from build123d import *

# Parameters (mm, degrees)
SKETCH_1_R      = 2
EXTRUDE_1_DEPTH = 3


with BuildPart() as part:
    # 草图1 → 凸台-拉伸1 (new body)
    with BuildSketch(Plane.XY):
        with BuildLine():
            Line((47.983882687, 10.173144913), (30.663374611, 20.173144913))
            ThreePointArc((30.663374611, 20.173144913), (-1.771986525, 14.862979702), (-28.921960456, 33.386732619))
            Line((-28.921960456, 33.386732619), (-48.921960456, 33.386732619))
            Line((-48.921960456, 33.386732619), (-48.921960456, -16.613267381))
            Line((-48.921960456, -16.613267381), (-28.921960456, -16.613267381))
            ThreePointArc((-28.921960456, -16.613267381), (-22.343103236, -10.961079821), (-13.724464148, -11.93455135))
            Line((-13.724464148, -11.93455135), (-5.391960456, -16.745324599))
            Line((-5.391960456, -16.745324599), (-5.391960456, -49.292329983))
            Line((-5.391960456, -49.292329983), (14.608039544, -49.292329983))
            Line((14.608039544, -49.292329983), (14.608039544, -36.952584021))
            ThreePointArc((14.608039544, -36.952584021), (17.108039544, -32.622457002), (22.108039544, -32.622457002))
            Line((22.108039544, -32.622457002), (31.644136725, -38.128125276))
            Line((31.644136725, -38.128125276), (41.644136725, -20.8076172))
            ThreePointArc((41.644136725, -20.8076172), (42.599829652, -4.864137572), (47.983882687, 10.173144913))
        make_face()
        with Locations((-38.921960456, 23.386732619)):
            Circle(SKETCH_1_R, mode=Mode.SUBTRACT)
        with Locations((-38.921960456, 8.386732619)):
            Circle(SKETCH_1_R, mode=Mode.SUBTRACT)
        with Locations((-38.921960456, -6.613267381)):
            Circle(SKETCH_1_R, mode=Mode.SUBTRACT)
        with Locations((-15.317387503, 0.532128762)):
            Circle(SKETCH_1_R, mode=Mode.SUBTRACT)
        with Locations((34.323628649, 6.512890875)):
            Circle(SKETCH_1_R, mode=Mode.SUBTRACT)
        with Locations((29.323628649, -2.147363162)):
            Circle(SKETCH_1_R, mode=Mode.SUBTRACT)
        with Locations((19.323628649, -19.467871238)):
            Circle(SKETCH_1_R, mode=Mode.SUBTRACT)
        with Locations((27.983882687, -24.467871238)):
            Circle(SKETCH_1_R, mode=Mode.SUBTRACT)
        with Locations((4.608039544, -31.292329983)):
            Circle(SKETCH_1_R, mode=Mode.SUBTRACT)
        with Locations((4.608039544, -41.292329983)):
            Circle(SKETCH_1_R, mode=Mode.SUBTRACT)
    extrude(amount=EXTRUDE_1_DEPTH)


solid = part.part
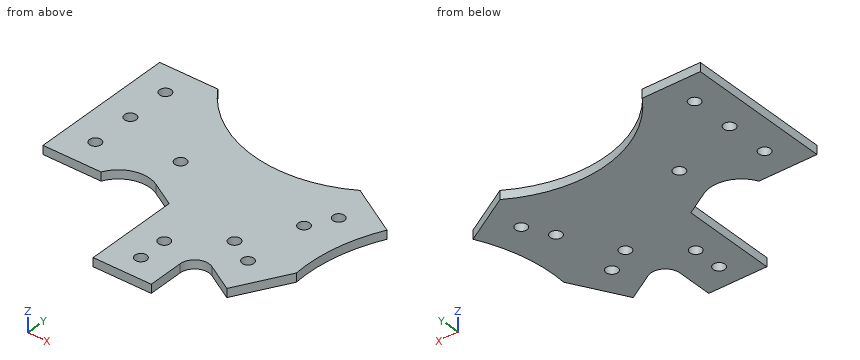
Source: CAD feature listing. Evaluate the final solid. Frame: model axes, mm. Coordinates: 2 decimals unless noted, no trailing zeros. Loops run counter-clockwise (first coordinate to the right, second up) from the corner with the lowest first, then second, coordinate; pieces in that order, holes last. Notation, with made-up numbers: M 61,4 L 67,4 A19 cw 67,39 Z; hole C -13,20 d4. An arc over 180 degrees is marked long. Answer in a Markdown table with one row per item.
Q1. Section B-B on z = 0.7. State how many separate pieces and enclosed holes the cut face has, plus the area to 3 significant figures.
Answers below:
| item | result |
|---|---|
| separate pieces | 1 |
| enclosed holes | 10 |
| area | 4,370 mm^2 |
Q2. Section A-A on y = 16. Return the cut outline in (x, z).
Answers below:
| item | result |
|---|---|
| outline | M -48.92,0 L -5.93,0 L -5.93,3 L -48.92,3 Z; M 21.55,0 L 37.89,0 L 37.89,3 L 21.55,3 Z |
Q3. Ray query, probe 1 along Y at (x, z) = (28, 1.5); probe 2 along Y at (x, z) = (28.5, 2.6); probe 3 along X at (y, z) = (-0.5, 1.55). Return the intervals inside material, ascending. Write a range as from..to.
Answers below:
| item | result |
|---|---|
| probe 1 | y = -36.02..-26.47, -22.47..-3.65, -0.65..18.69 |
| probe 2 | y = -36.31..-26.4, -22.54..-3.97, -0.32..18.95 |
| probe 3 | x = -48.92..-17.03, -13.6..28.19, 30.46..43.68 |
Q4. Section D-D on x = 0. Return the cut outline in (y, z).
Answers below:
| item | result |
|---|---|
| outline | M -49.29,0 L 14.51,0 L 14.51,3 L -49.29,3 Z |
Q5. First-contact query: pin 1 (4.5 mm diameter, centred on x = 19.32, y = -19.47, fed in from -Z); pin 2 (1.5 mm diameter, centred on x = 32.5, z = 2, fed in from -Y); pin 3 (1.5 mm diameter, centred on y = -45.5, z = 1.5, fed in from +X); pin 4 (3.5 mm diameter, centred on x = 4.61, y = -41.29, fed in from -Z). Flat tips, straight axial feed; report the tip coordinate or a pass-through.
Answers below:
| item | result |
|---|---|
| pin 1 | stops at z = 0 |
| pin 2 | stops at y = -37.94 |
| pin 3 | stops at x = 14.61 |
| pin 4 | passes through |
Q6. Section C-C on x = -31. Return the cut outline in (y, z), plus the area to 3 significant figures.
Answers below:
| item | result |
|---|---|
| outline | M -16.61,0 L 33.39,0 L 33.39,3 L -16.61,3 Z |
| area | 150 mm^2 |
